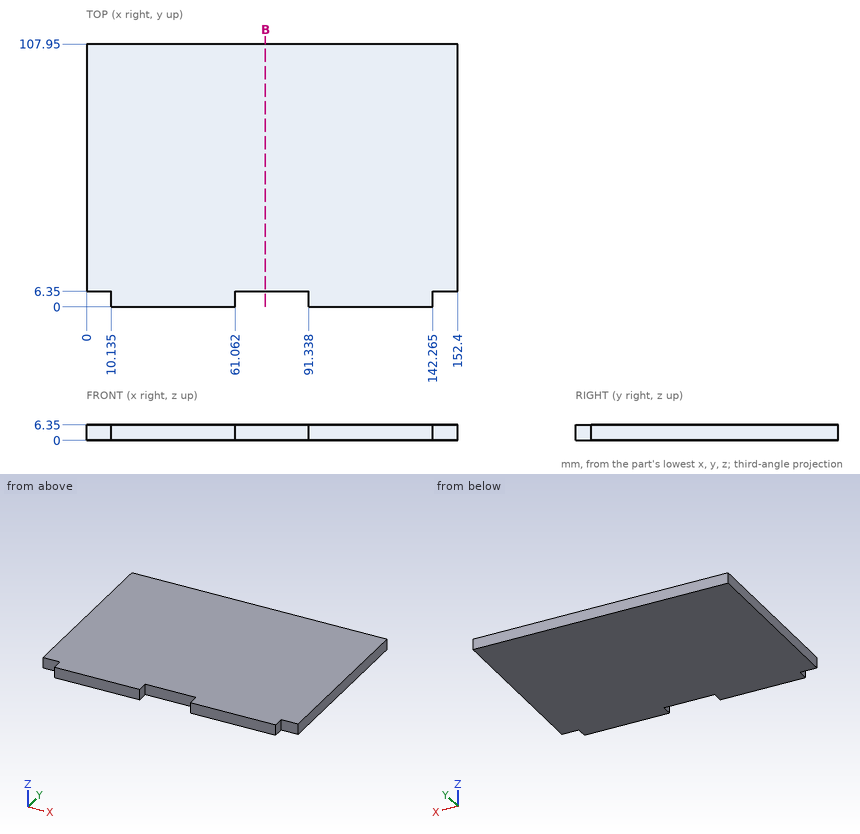
Design review of the part shown in the three views and the two pictorial views. Dimensions are in mm from the part's minimum x, y and z. Round coordinates to 2 decimals unless told otherwise and drop trailing zeros. Order: outer loops, then holes, each group sorted by start corner. A loop starts at its lowest first (then second) coordinate and runs counter-clockwise, first axis right, second up.
Item 1: Add section B-B, the plane x = 73.5. State the section outline as (y, z) points, and give its area (3 significant figures).
Working result:
outline: (6.35, 0) - (107.95, 0) - (107.95, 6.35) - (6.35, 6.35) - close
area: 645 mm2
Item 2: To check wall thickness, follow probe 1 along Y at (x, z) = (62, 5.75). State the ranges of the line that lie inside material, in increasing order.
Working result:
probe 1: y = 6.35 to 107.95
Item 3: For pin 1 (3 mm diameter, centred on y = 3, z = 3.5, fed in from +X) (3 decimals); pin 2 (1.9 mm diameter, centred on y = 4, z = 2, fed in from -X) (3 decimals); pin 3 (1.9 mm diameter, centred on x = 71.5, z = 4, fed in from -Y), all flat-tipped, find the tip position at first contact; note any pin that passes through.
Working result:
pin 1: stops at x = 142.265
pin 2: stops at x = 10.135
pin 3: stops at y = 6.35
